from build123d import *

# Parameters (mm, degrees)
SKETCH2_R           = 3.84
BOSS_EXTRUDE1_DEPTH = 0.387623957
SKETCH3_R           = 3.84
BOSS_EXTRUDE2_DEPTH = 0.092376043
BOSS_EXTRUDE2_TAPER = -60.000000004
SKETCH4_R           = 4
BOSS_EXTRUDE3_DEPTH = 14.52
SKETCH5_R           = 2.3865
BOSS_EXTRUDE4_DEPTH = 1.25
SKETCH6_R           = 2.3865
BOSS_EXTRUDE5_DEPTH = 0.6135
BOSS_EXTRUDE5_TAPER = -45
SKETCH7_R           = 3
BOSS_EXTRUDE6_DEPTH = 7.1365
CUT_EXTRUDE1_DEPTH  = 3
CHAMFER1_SIZE       = 0.6135
FILLET1_R           = 0.261


with BuildPart() as part:
    # Sketch1 → Revolve1 (revolve)
    with BuildSketch(Plane(origin=(0, 0, 0), x_dir=(-1, 0, 0), z_dir=(0, 0, -1))):
        with BuildLine():
            Line((0, 6.5), (0, 0))
            Line((0, 0), (6, 0))
            Line((6, 0), (6, 6.5))
            Line((6, 6.5), (3.3, 6.5))
            ThreePointArc((3.3, 6.5), (3, 6.2), (2.7, 6.5))
            Line((2.7, 6.5), (0, 6.5))
        make_face()
    revolve(axis=Axis((0, 0, 0), (-1, 0, 0)))

    # Sketch2 → Boss-Extrude1 (add)
    with BuildSketch(Plane(origin=(0, 0, 0), x_dir=(0, 0, -1), z_dir=(1, 0, 0))):
        Circle(SKETCH2_R)
    extrude(amount=BOSS_EXTRUDE1_DEPTH)

    # Sketch3 → Boss-Extrude2 (add)
    with BuildSketch(Plane(origin=(0.387623957, 0, 0), x_dir=(0, 0, -1), z_dir=(1, 0, 0))):
        Circle(SKETCH3_R)
    extrude(amount=BOSS_EXTRUDE2_DEPTH, taper=BOSS_EXTRUDE2_TAPER)

    # Sketch4 → Boss-Extrude3 (add)
    with BuildSketch(Plane(origin=(0.48, 0, 0), x_dir=(0, 0, -1), z_dir=(1, 0, 0))):
        Circle(SKETCH4_R)
    extrude(amount=BOSS_EXTRUDE3_DEPTH)

    # Sketch5 → Boss-Extrude4 (add)
    with BuildSketch(Plane(origin=(15, 0, 0), x_dir=(0, 0, -1), z_dir=(1, 0, 0))):
        Circle(SKETCH5_R)
    extrude(amount=BOSS_EXTRUDE4_DEPTH)

    # Sketch6 → Boss-Extrude5 (add)
    with BuildSketch(Plane(origin=(16.25, 0, 0), x_dir=(0, 0, -1), z_dir=(1, 0, 0))):
        Circle(SKETCH6_R)
    extrude(amount=BOSS_EXTRUDE5_DEPTH, taper=BOSS_EXTRUDE5_TAPER)

    # Sketch7 → Boss-Extrude6 (add)
    with BuildSketch(Plane(origin=(16.8635, 0, 0), x_dir=(0, 0, -1), z_dir=(1, 0, 0))):
        Circle(SKETCH7_R)
    extrude(amount=BOSS_EXTRUDE6_DEPTH)

    # Sketch8 → Cut-Extrude1 (cut)
    with BuildSketch(Plane.ZY.offset(6)):
        Polygon((2.5, -1.443375673), (2.5, 1.443375673), (0, 2.886751346), (-2.5, 1.443375673), (-2.5, -1.443375673), (0, -2.886751346), align=None)
    extrude(amount=-CUT_EXTRUDE1_DEPTH, mode=Mode.SUBTRACT)

    # Sketch9 → Cut-Revolve1 (revolve, cut)
    with BuildSketch(Plane.XY):
        Polygon((-3, 2.4), (-3, 0), (-1.614359354, 0), align=None)
    revolve(axis=Axis((-3, 0, 0), (1, 0, 0)), mode=Mode.SUBTRACT)

    # Chamfer1
    chamfer1_edges = [part.edges().sort_by_distance(p)[0] for p in [
        (24, 0, 3),
        (-6, -6.5, 0),
    ]]
    chamfer(chamfer1_edges, length=CHAMFER1_SIZE)

    # Fillet1
    fillet1_edges = [part.edges().sort_by_distance(p)[0] for p in [
        (0, 0, 3.84),
    ]]
    fillet(fillet1_edges, radius=FILLET1_R)


solid = part.part
Input: part model. Units: mm. Frame: model coordinates. A direction names the side the tool comes from. Give positions to 0.01 mm unless a question says otherwise; leave off trailing zeros. Loops run counter-clockwise (first coordinate to the right, second up) from the corner with the lowest first, then second, coordinate; pieces in that order, holes last. Notation, with made-up numbers: M -12,-36 L 14,-36 A14 cw 14,-18 Z; hole C 59,0.25 d5. An arc over 180 degrees is marked long. Use CSV: the item, a comma, the result in double quotes.
(1) Material intervals for L1, parallel to X at y = -0.75, z = -4.75; L2, parallel to Y at x = 0.25, z = 3; L3, parallel to X at y = -0.5, z = -3.25, sorted ascending. Write a range as [from, to].
Outcome:
L1,"x = [-6, 0]"
L2,"y = [-2.4, 2.4]"
L3,"x = [-6, 15]"
(2) Section B-B, the plane x = 8.5. Return loops of the section in (y, z), plus the area to 3 significant figures.
Outcome:
outline,"C 0,0 d8"
area,"50.3 mm²"
(3) Pin query (flat end, axial travel): P1, Ø1.5, axis at x = 8, z = -1.5, coming from the +Y side; P2, Ø2, axis at x = 14.5, y = -0.5, coming from the +Z side; P3, Ø3, axis at x = 12, y = -3.5, coming from the -Z side. Return the tip coordinate at first contact, or that it passes through.
Outcome:
P1,"stops at y = 3.93"
P2,"stops at z = 4"
P3,"stops at z = -3.46"
(4) Section A-A, the plane x = 22. Return loops of the section in (y, z), plus the area to 3 significant figures.
Outcome:
outline,"C 0,0 d6"
area,"28.3 mm²"
(5) Pull-direction query (Y, two-part tool) for faces 1 (the face through (-4.521, 2.175, -1.233)), 2 (the face through (-6, 0, 3)), 3 (the face through (-4.521, -2.155, -1.267)), 4 (the face through (20, 0, 3)); classes: pulls with the +Y half, pulls with the -Y half, needs draft (parallel to the pull), parting line crosses it, or undercut.
Outcome:
face 1,"undercut"
face 2,"needs draft"
face 3,"undercut"
face 4,"parting line crosses it"
(6) Set-up query: faces 5 (the face through (-4.521, 2.155, 1.267)), 6 (the face through (7.638, -3.905, 0.867)), 7 (the face through (15, -2, -2)). Return all of +Z, -Z, +X, -X, +Y, -Y with unobstructed straight access to the full face (end or side cutting, diameter ignored); none if empty.
Outcome:
face 5,"-X"
face 6,"+X"
face 7,"none"
